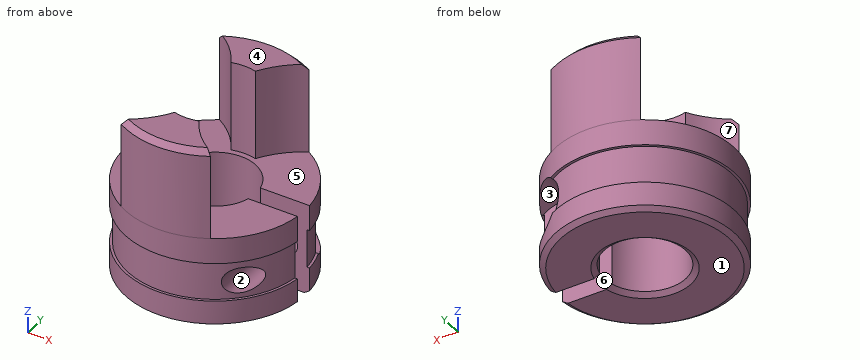
from build123d import *
from OCP.BRepFilletAPI import BRepFilletAPI_MakeChamfer

# Parameters (mm, degrees)
BOSS_EXTRUDE1_START     = -3.937
SKETCH1_R               = 6.985
BOSS_EXTRUDE1_DEPTH     = 7.112
CUT_EXTRUDE10_START     = -2
SKETCH25_R              = 6.985
SKETCH25_R_2            = 6.785
CUT_EXTRUDE10_DEPTH     = 3
BOSS_EXTRUDE2_DEPTH     = 7
CIRPATTERN1_COUNT       = 2
CUT_EXTRUDE5_DEPTH      = 15.820959854
CUT_EXTRUDE5_DEPTH_BACK = 15.820959854
SKETCH15_R              = 3.175
CHAMFER1_SIZE           = 0.2794
CHAMFER1_SIZE2          = 0.414227535
SKETCH19_R              = 2.154
CUT_EXTRUDE6_DEPTH      = 17.15041344
SKETCH23_W              = 6.985
SKETCH23_H              = 1.5
CUT_EXTRUDE9_DEPTH      = 15.820959948
CHAMFER6_SIZE           = 0.4191


with BuildPart() as part:
    # Sketch1 → Boss-Extrude1 (new body)
    with BuildSketch(Plane.XY.offset(BOSS_EXTRUDE1_START)):
        Circle(SKETCH1_R)
    extrude(amount=-BOSS_EXTRUDE1_DEPTH)

    # Sketch25 → Cut-Extrude10 (cut)
    with BuildSketch(Plane.XY.offset(-3.937).offset(CUT_EXTRUDE10_START)):
        Circle(SKETCH25_R)
        Circle(SKETCH25_R_2, mode=Mode.SUBTRACT)
    extrude(amount=-CUT_EXTRUDE10_DEPTH, mode=Mode.SUBTRACT)

    # Sketch2 → Boss-Extrude2 (add)
    with BuildSketch(Plane.XY.offset(-3.937)):
        with BuildLine():
            ThreePointArc((-3.5, -6.044851115), (0, -6.985), (3.5, -6.044851115))
            ThreePointArc((3.5, -6.044851115), (2.056519165, -4.92606064), (0.951562077, -3.471963366))
            ThreePointArc((0.951562077, -3.471963366), (0, -3.6), (-0.951562077, -3.471963366))
            ThreePointArc((-0.951562077, -3.471963366), (-2.056519165, -4.92606064), (-3.5, -6.044851115))
        make_face()
    boss_extrude2 = extrude(amount=BOSS_EXTRUDE2_DEPTH)

    # CirPattern1: Boss-Extrude2 ×2 about axis
    cirpattern1_axis = Axis((0, 0, 0), (0, 0, 1))
    for i in range(1, CIRPATTERN1_COUNT):
        add(boss_extrude2.rotate(cirpattern1_axis, i * 360 / CIRPATTERN1_COUNT))

    # Sketch15 → Cut-Extrude5 (cut, two sides: drawn at the far end of the back side and taken through both)
    with BuildSketch(Plane.XY.offset(-CUT_EXTRUDE5_DEPTH_BACK)):
        Circle(SKETCH15_R)
    extrude(amount=CUT_EXTRUDE5_DEPTH + CUT_EXTRUDE5_DEPTH_BACK, mode=Mode.SUBTRACT)

    # Chamfer1: one chamfer whose edges measure the first distance from different faces: ONE call of the kernel's chamfer builder (chamfer() names one face for all edges)
    chamfer1_edges_1 = [part.edges().sort_by_distance(p)[0] for p in [
        (-3.175, 0, -11.049),
    ]]
    chamfer1_side_1 = [part.faces().sort_by_distance(p)[0] for p in [
        (-3.175, 0, -7.493),
    ]]
    chamfer1_edges_2 = [part.edges().sort_by_distance(p)[0] for p in [
        (-6.985, 0, -11.049),
    ]]
    chamfer1_side_2 = [part.faces().sort_by_distance(p)[0] for p in [
        (-6.985, 0, -9.993),
    ]]
    chamfer1 = BRepFilletAPI_MakeChamfer(part.part.solid().wrapped)
    for e in chamfer1_edges_1:
        chamfer1.Add(CHAMFER1_SIZE, CHAMFER1_SIZE2, e.wrapped, chamfer1_side_1[0].wrapped)  # the first distance lies on this face
    for e in chamfer1_edges_2:
        chamfer1.Add(CHAMFER1_SIZE, CHAMFER1_SIZE2, e.wrapped, chamfer1_side_2[0].wrapped)  # the first distance lies on this face
    add(Compound.cast(chamfer1.Shape()), mode=Mode.REPLACE)

    # Sketch17 → Cut-Revolve1 (revolve, cut)
    with BuildSketch(Plane(origin=(0, 0, -7.549), x_dir=(-1, 0, 0), z_dir=(0, 0, -1)), mode=Mode.PRIVATE) as cut_revolve1_sk:
        Polygon((-6, 2.5), (-6, -7.201139233), (-5, -7.201139233), (-5, 4.499600677), (-5, 8.2375), (-6.9, 8.2375), (-6.9, 4.499600677), (-6.9, 2.5), align=None)
    revolve(cut_revolve1_sk.sketch.rotate(Axis((5, 4.499600677, -7.549), (0, -1, 0)), 180), axis=Axis((5, 4.499600677, -7.549), (0, -1, 0)), mode=Mode.SUBTRACT)

    # Sketch19 → Cut-Extrude6 (cut, through all)
    with BuildSketch(Plane(origin=(0, 2.5, 0), x_dir=(1, 0, 0), z_dir=(0, 1, 0))):
        with Locations((5, 7.549)):
            Circle(SKETCH19_R)
    extrude(amount=CUT_EXTRUDE6_DEPTH, mode=Mode.SUBTRACT)

    # Sketch23 → Cut-Extrude9 (cut, through all)
    with BuildSketch(Plane.XY):
        with Locations((3.4925, 0)):
            Rectangle(SKETCH23_W, SKETCH23_H)
    extrude(amount=-CUT_EXTRUDE9_DEPTH, mode=Mode.SUBTRACT)

    # Chamfer6
    chamfer6_edges = [part.edges().sort_by_distance(p)[0] for p in [
        (0, -6.985, 3.063),
        (0, 6.985, 3.063),
    ]]
    chamfer(chamfer6_edges, length=CHAMFER6_SIZE)


solid = part.part
The model under review builds one solid part; all positions refer to its coordinate system, in mm. Face numbers are marked on the shaded views. A direction names the side the tool comes from. Round coordinates to 2 decimals unless told otherwise and drop trailing zeros. Order: outer loops, then holes, each group sorted by start corner. A loop starts at its lowest first (then second) coordinate and runs counter-clockwise, first axis right, second up. Notation, with made-up numbers: (-38, -35.75) -> (0, -35.75) arc R19 ccw to (0, -4.75) -> close; hole circle Ø6 at (49, -23). An arc over 180 degrees is marked (long way). Return JSON: item names as keys, results as strings.
1. Take a section at C-C (y = 0). Write out the cut boundary in (x, z) (3 decimals), then the cut area to 3 significant figures.
Answer block:
{"outline": "(-6.985, -10.77) -> (-6.571, -11.049) -> (-3.589, -11.049) -> (-3.175, -10.77) -> (-3.175, -3.937) -> (-6.985, -3.937) -> (-6.985, -5.937) -> (-6.785, -5.937) -> (-6.785, -8.937) -> (-6.985, -8.937) -> close", "area": "26.4 mm²"}
2. Take a section at B-B (z = -0.75). Write out the cut boundary in (x, y) (3 decimals).
Answer block:
{"outline": "(-3.5, -6.045) arc R6.985 ccw to (3.5, -6.045) arc R7 cw to (0.952, -3.472) arc R3.6 cw to (-0.952, -3.472) arc R7 cw to start; (-3.5, 6.045) arc R7 cw to (-0.952, 3.472) arc R3.6 cw to (0.952, 3.472) arc R7 cw to (3.5, 6.045) arc R6.985 ccw to start"}
3. For the marked faces 5, 6 and 7, list the 3-axis set-ups (+Z, -Z, +X, -X, +Y, -Y) from which the entire face can be reached by the end or side of a thin tool; tool diameter is ignored.
Answer block:
{"face 5": "+Z", "face 6": "+Z, -Z, +X", "face 7": "+Z, -X"}
4. Take a section at A-A (x = 0). Write out the cut boundary in (y, z) (3 decimals), then the cut area to 4 significant figures.
Answer block:
{"outline": "(-6.985, -10.77) -> (-6.571, -11.049) -> (-3.589, -11.049) -> (-3.175, -10.77) -> (-3.175, -3.937) -> (-3.6, -3.937) -> (-3.6, 3.063) -> (-6.566, 3.063) -> (-6.985, 2.644) -> (-6.985, -5.937) -> (-6.785, -5.937) -> (-6.785, -8.937) -> (-6.985, -8.937) -> close; (3.175, -10.77) -> (3.589, -11.049) -> (6.571, -11.049) -> (6.985, -10.77) -> (6.985, -8.937) -> (6.785, -8.937) -> (6.785, -5.937) -> (6.985, -5.937) -> (6.985, 2.644) -> (6.566, 3.063) -> (3.6, 3.063) -> (3.6, -3.937) -> (3.175, -3.937) -> close", "area": "100.0 mm²"}
5. The part is to be moulded in two halves that separate along Z. For the marked faces 1, 2, 3 and 4, say which applies: +Z half, -Z half, draft (parallel to the pull), parting line (faces both ways), or undercut.
Answer block:
{"face 1": "-Z half", "face 2": "undercut", "face 3": "undercut", "face 4": "+Z half"}
6. Take a section at D-D (y = -2). State how many separate pieces and enclosed holes the cut face has, then the cut area to 3 significant figures.
Answer block:
{"separate pieces": "2", "enclosed holes": "1", "area": "55.5 mm²"}
7. Insertion check: P1, Ø1.9, axis at x = 5.5, z = -7.5, coming from the +Y side; P2, Ø1.5, axis at x = -2, z = -4.5, coming from the -Y side; P3, Ø3, axis at x = -2, z = -4, coming from the +Y side. Each pin has a flat end and moves straight along its axis. Give the tip position at first contact, or say it passes through.
Answer block:
{"P1": "stops at y = 2.5", "P2": "stops at y = -6.87", "P3": "stops at y = 6.97"}
8. For L1, parallel to Z at x = 5, y = 1.1; L2, parallel to Y at x = 0.25, z = -3.75; L3, parallel to Z at x = 5, y = 3 (3 decimals), list the stretches that pass through material, from the lowest coordinate up. Write a range as [from, to].
Answer block:
{"L1": "z = [-11.05, -8.55], [-6.55, -3.94]", "L2": "y = [-6.98, -3.59], [3.59, 6.98]", "L3": "z = [-11.049, -9.703], [-5.395, -3.937]"}
